CAD build for the part. Positions are in the model's coordinates, mm. A direction names the side the tool comes from. Coordinates: 2 decimals unless noted, no trailing zeros. Loops run counter-clockwise (first coordinate to the right, second up) from the corner with the lowest first, then second, coordinate; pieces in that order, holes last. Notation, with made-up numbers: (50, 74.5) -> (73, 74.5) arc R11 ccw to (73, 87.5) -> close; hole circle Ø6 at (38.5, 6.5). An arc over 180 degrees is marked (long way). Answer as CSV lines item,"result". Start each with the question number.
from build123d import *

# Parameters (mm, degrees)
F1_DEPTH = 4
F3_DEPTH = 2


with BuildPart() as f1:
    # F0 (on Top) → F1 (new body)
    with BuildSketch(Plane.XY):
        with BuildLine():
            ThreePointArc((18.939283, 23.590199), (-25.962329, -14.538319), (29.925106, 4.077085))
            ThreePointArc((29.925106, 4.077085), (36.258822, 20.491997), (18.939283, 23.590199))
        make_face()
        with BuildLine():
            ThreePointArc((22.029397, 20.736062), (32.635662, 18.452168), (29.087509, 8.199382))
            ThreePointArc((29.087509, 8.199382), (26.321098, 14.897089), (22.029397, 20.736062))
        make_face(mode=Mode.SUBTRACT)
    extrude(amount=F1_DEPTH)

    # F2 (on face) → F3 (join)
    with BuildSketch(Plane.XY.offset(4)):
        Polygon((-11.189207, 17.327955), (-18.506745, -8.068205), (-7.962489, -8.2658), (-1.145528, 17.327955), align=None)
    extrude(amount=F3_DEPTH)


solid = f1.part
Item 1: Wall check: probe 1 along Z at (x, y) = (17.5, 8.5); probe 2 along X at (y, z) = (-0.5, 3.9); probe 3 along X at (y, z) = (8.5, 3.05). Give the ranges that are in metal, low to high.
Item 2: Two-plate mould, pull along X, no slides. Class faces 4 (the face through (32.55, 18.6, 1.97)), 5 (the face through (-4.602, 4.352, 4.986)), 6 (the face through (-14.8, 4.8, 5)), 7 (the face through (-10, 5, 6)): pulls with the +X half, pulls with the -X half, needs draft (parallel to the pull), parting line crosses it, or undercut.
Item 3: Saw through at D-D (z = 3.25). Write the cut outline in (x, y).
Item 4: Saw through at A-A (x = -12). Write the cut outline in (y, z).
Item 5: Which spindle directions (+Z, -Z, +X, -X, +Y, -Y) get a long thin tool onto all of the face, cutting with end or side? Do faces 1 (the face through (26.37, 14.81, 1.97)), 2 (the face through (3, 1, 0)), 3 (the face through (-6, 17.328, 5)). Say none if no direction does.
Item 6: Saw through at C-C (y = -1.5). Write the cut outline in (x, z).
Item 7: Flat gauge pins, fed straight in: pin 1 Ø1.5 at (y, z) = (21.5, 2.5) entering from -X; pin 2 Ø1 at (x, z) = (-5.5, 5.5) entering from +Y; pin 3 Ø1 at (y, z) = (11.5, 4) entering from -X. Where does each tip first touch, or does it go through?
Item 8: Saw through at B-B (y = 9). Write the cut outline in (x, z), plus the area to 3 significant figures.
Geometry check:
1,probe 1,"0 to 4"
1,probe 2,"-29.81 to 30.17"
1,probe 3,"-28.64 to 29, 29.73 to 35.76"
2,face 4,"undercut"
2,face 5,"pulls with the +X half"
2,face 6,"pulls with the -X half"
2,face 7,"needs draft"
3,outline,"(18.94, 23.59) arc R30 ccw (long way) to (29.93, 4.08) arc R11.4 ccw (long way) to start; hole (22.03, 20.74) arc R30 cw to (29.09, 8.2) arc R7.25 ccw (long way) to start"
4,outline,"(-27.24, 0) -> (27.6, 0) -> (27.6, 4) -> (14.51, 4) -> (14.51, 6) -> (-8.19, 6) -> (-8.19, 4) -> (-27.24, 4) -> close"
5,face 1,"+Z, -Z"
5,face 2,"-Z, +X, -X, +Y, -Y"
5,face 3,"+Z, +X, -X, +Y"
6,outline,"(-29.77, 0) -> (30.13, 0) -> (30.13, 4) -> (-6.16, 4) -> (-6.16, 6) -> (-16.61, 6) -> (-16.61, 4) -> (-29.77, 4) -> close"
7,pin 1,"x = -21.66"
7,pin 2,"y = 17.33"
7,pin 3,"x = -27.8"
8,outline,"(-28.49, 0) -> (28.85, 0) -> (28.85, 4) -> (-3.36, 4) -> (-3.36, 6) -> (-13.59, 6) -> (-13.59, 4) -> (-28.49, 4) -> close; (30.53, 0) -> (36.08, 0) -> (36.08, 4) -> (30.53, 4) -> close"
8,area,"272 mm2"
